Read the model definition and answer for the solid it produces. Units are mm, in the model's axes. Face numbers are marked on the shaded views. A direction names the side the tool comes from. Give positions to 0.01 mm unless a question says otherwise; leave off trailing zeros. Loops run counter-clockwise (first coordinate to the right, second up) from the corner with the lowest first, then second, coordinate; pieces in that order, holes last. Notation, with made-up numbers: (42, 49) - (81, 49) arc R17 ccw to (81, 82) - close; hole circle Ø9 at (86, -29). An arc over 180 degrees is marked (long way). Write item = value, one per line.
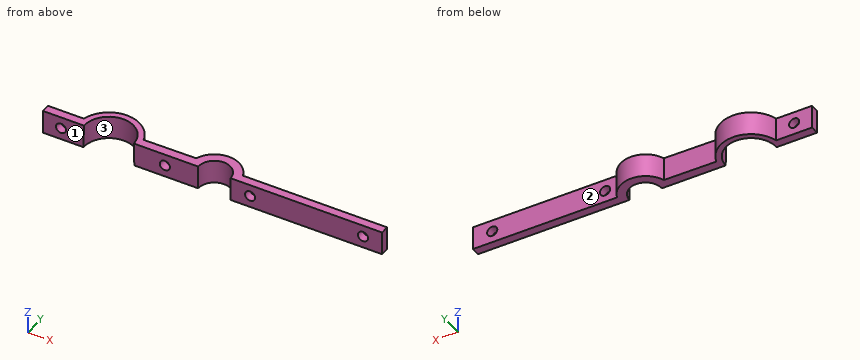
Autodesk Fusion 360 part; units mm, degrees
sketch "Sketch1" plane through (0, 0, 0) normal (0, 0, 1) x (1, 0, 0)
  circle A0 centre (-43.925, 0) radius 12.925
  circle A1 centre (0, 0) radius 10.5
  circle A2 centre (0, 0) radius 6.75
  line L0 (9.8995, 3.5) -> (69.8995, 3.5)
  line L1 (69.8995, 3.5) -> (69.8995, -3.5)
  line L2 (69.8995, -3.5) -> (9.8995, -3.5)
  line L3 (-31.5162, 3.6163) -> (-9.7806, 3.8197)
  line L4 (-31.4507, -3.3834) -> (-10.006, -3.1827)
  line L5 (-56.3671, 3.5) -> (-71.3671, 3.5)
  line L6 (-71.3671, 3.5) -> (-71.3671, -3.5)
  line L7 (-71.3671, -3.5) -> (-56.3671, -3.5)
  line L8 (-43.925, 0) -> (0, 0) construction
  dimension "d1" = 3.5
  dimension "d2" = 3.5
  dimension "d3" = 3.5
  dimension "d4" = 3.5
  dimension "d5" = 3.5
  dimension "d6" = 3.5
  dimension "d7" = 43.925
  dimension "d8" = 60
  dimension "d9" = 15
  dimension "d19" = 25.85
  dimension "d20" = 21
  dimension "d21" = 13.5
extrude "Extrude1" add sketch "Sketch1" along normal mid plane 10
sketch "Sketch4" plane through (0, 3.5, 0) normal (0, 1, 0) x (-1, 0, 0)
  line L0 (71.3671, -5) -> (71.3671, 5)
  line L1 (71.3671, 5) -> (56.3671, 5)
  line L2 (56.3671, 5) -> (56.3671, -5)
  line L3 (56.3671, -5) -> (71.3671, -5)
  circle A0 centre (63.8671, 0) radius 2.125
  line L4 (31.5162, -5) -> (9.7806, -5)
  line L5 (31.5162, 5) -> (31.5162, -5)
  line L6 (9.7806, -5) -> (9.7806, 5)
  dimension "d25" = 4.25
  dimension "d27" = 5
  dimension "d31" = 7.5
  dimension "d32" = 7.5
extrude "Extrude4" cut sketch "Sketch4" along normal up to surface contours A0 end surface through (-31.4507, -3.3834, 0) normal (0.009359, -0.999956, 0) offset 0
sketch "Sketch5" plane through (-0.0366, 3.9109, 0) normal (-0.0094, 1, 0) x (0, 0, 1)
  line L0 (-5, -31.481) -> (5, -31.481)
  line L1 (5, -31.481) -> (5, -9.7444)
  line L2 (5, -9.7444) -> (-5, -9.7444)
  line L3 (-5, -9.7444) -> (-5, -31.481)
  circle A0 centre (0, -20.613) radius 2.125
  dimension "d35" = 4.25
  dimension "d36" = 10.868
  dimension "d37" = 10.8686
  dimension "d38" = 5
extrude "Extrude5" cut sketch "Sketch5" against normal up to surface (7 mm away) contours A0
sketch "Sketch6" plane through (0, 3.5, 0) normal (0, 1, 0) x (-1, 0, 0)
  line L0 (-9.8995, -5) -> (-9.8995, 5)
  line L1 (-9.8995, 5) -> (-69.8995, 5)
  line L2 (-69.8995, 5) -> (-69.8995, -5)
  line L3 (-69.8995, -5) -> (-9.8995, -5)
sketch "Sketch7" plane through (0, 3.5, 0) normal (0, 1, 0) x (-1, 0, 0)
  line L0 (-9.8995, -5) -> (-9.8995, 5) construction
  line L1 (-9.8995, 5) -> (-69.8995, 5) construction
  line L2 (-69.8995, 5) -> (-69.8995, -5) construction
  line L3 (-69.8995, -5) -> (-9.8995, -5) construction
  line L4 (-69.8995, 0) -> (-9.8995, 0) construction
  circle A0 centre (-61.8995, 0) radius 2.125
  circle A1 centre (-14.8995, 0) radius 2.125
  dimension "d41" = 4.25
  dimension "d42" = 4.25
  dimension "d43" = 8
  dimension "d44" = 5
extrude "Extrude6" cut sketch "Sketch7" against normal up to surface (7 mm away)
sketch "Sketch8" plane through (0, 0, 5) normal (0, 0, 1) x (1, 0, 0)
  circle A0 centre (0, 0) radius 6.75
  arc A1 (-31.5162, 3.6163) -> (-56.3671, 3.5) centre (-43.925, 0) ccw
  line L0 (-56.3671, 3.5) -> (-71.3671, 3.5)
  line L1 (-71.3671, 3.5) -> (-71.3671, -3.5)
  line L2 (-71.3671, -3.5) -> (-56.3671, -3.5)
  arc A2 (-56.3671, -3.5) -> (-31.4507, -3.3834) centre (-43.925, 0) ccw
  line L3 (-31.4507, -3.3834) -> (-10.006, -3.1827)
  arc A3 (-10.006, -3.1827) -> (9.8995, -3.5) centre (0, 0) ccw
  line L4 (9.8995, -3.5) -> (69.8995, -3.5)
  line L5 (69.8995, -3.5) -> (69.8995, 3.5)
  line L6 (69.8995, 3.5) -> (9.8995, 3.5)
  arc A4 (9.8995, 3.5) -> (-9.7806, 3.8197) centre (0, 0) ccw
  line L7 (-9.7806, 3.8197) -> (-31.5162, 3.6163)
  circle A5 centre (-43.925, 0) radius 12.925 construction
  circle A6 centre (-43.925, 0) radius 10.37
  dimension "d49" = 20.74
sketch "Sketch9" plane through (0, 0, -5) normal (0, 0, -1) x (-1, 0, 0)
  circle A0 centre (0, 0) radius 6.75
  arc A1 (56.3671, 3.5) -> (31.5162, 3.6163) centre (43.925, 0) ccw
  line L0 (31.5162, 3.6163) -> (9.7806, 3.8197)
  arc A2 (9.7806, 3.8197) -> (-9.8995, 3.5) centre (0, 0) ccw
  line L1 (-9.8995, 3.5) -> (-69.8995, 3.5)
  line L2 (-69.8995, 3.5) -> (-69.8995, -3.5)
  line L3 (-69.8995, -3.5) -> (-9.8995, -3.5)
  arc A3 (-9.8995, -3.5) -> (10.006, -3.1827) centre (0, 0) ccw
  line L4 (10.006, -3.1827) -> (31.4507, -3.3834)
  arc A4 (31.4507, -3.3834) -> (56.3671, -3.5) centre (43.925, 0) ccw
  line L5 (56.3671, -3.5) -> (71.3671, -3.5)
  line L6 (71.3671, -3.5) -> (71.3671, 3.5)
  line L7 (71.3671, 3.5) -> (56.3671, 3.5)
  circle A5 centre (43.925, 0) radius 12.925 construction
  circle A6 centre (43.925, 0) radius 10.6
  dimension "d50" = 21.2
loft "Loft1" cut profiles "Sketch8", "Sketch9" section 1 contours A6 section 2 contours A6
sketch "Sketch3" plane through (0, 0, 0) normal (0, 1, 0) x (1, 0, 0)
  line L0 (-71.3671, 5) -> (-71.3671, -5)
  line L1 (-71.3671, -5) -> (-56.3671, -5)
  line L2 (-56.3671, -5) -> (-56.3671, 5)
  line L3 (-56.3671, 5) -> (-71.3671, 5)
  line L4 (9.8995, 5) -> (9.8995, -5)
  line L5 (9.8995, -5) -> (69.8995, -5)
  line L6 (69.8995, -5) -> (69.8995, 5)
  line L7 (69.8995, 5) -> (9.8995, 5)
  line L8 (-71.3671, 5) -> (69.8995, 5)
  line L9 (69.8995, 5) -> (69.8995, -5)
  line L10 (69.8995, -5) -> (-71.3671, -5)
  line L11 (-71.3671, -5) -> (-71.3671, 5)
  circle A0 centre (-63.8671, 0) radius 2.125
  circle A1 centre (14.8995, 0) radius 2.125
  circle A2 centre (61.8995, 0) radius 2.125
extrude "Extrude3" cut sketch "Sketch3" against normal blind 20 contours L0 L1 L2 L3 L8 L10 L11 | L2 L4 L8 L10 | L4 L5 L6 L7 L8 L9 L10 | A0 | A1 | A2
equation "d2 = d1"
equation "d3 = d1"
equation "d4 = d1"
equation "d5 = d1"
equation "d6 = d1"
equation "d42 = d41"
1) A cutting plane is placed at B-B on x = 30.5. Determine the outline of the cut face in (y, z).
Output:
outline = (0, -5) - (3.5, -5) - (3.5, 5) - (0, 5) - close
2) A cutting plane is placed at D-D on x = 0. Determine the outline of the cut face in (y, z).
Output:
outline = (6.75, -5) - (10.5, -5) - (10.5, 5) - (6.75, 5) - close
3) A tool of negligible diameter and unlimited length cuts with its end or side. For the marked faces 1, 2 and 3, from which of +Z, -Z, +X, -X, +Y, -Y can it reach the whole face along a straight path? Write none if from no direction.
Output:
face_1 = +Z, -Z, +X, -X, -Y
face_2 = +Z, -Z, +X, +Y
face_3 = -Z, -Y
4) Find the intervals of material crossed by probe 1 along X at (y, z) = (7.5, 4.75); probe 2 along X at (y, z) = (7.75, -3.75); probe 3 along Y at (x, z) = (32, 1.5), in increasing order.
Output:
probe_1 = -54.45 to -51.09, -36.76 to -33.4, -7.35 to 7.35
probe_2 = -54.27 to -51.11, -36.74 to -33.58, -7.08 to 7.08
probe_3 = 0 to 3.5
5) Each of these flat-tipped pins is pushed along its axis until it touches: P1, Ø5, axis at x = -63.5, z = -1.5, coming from the +Y side; P2, Ø4, axis at x = -4.5, y = 4.5, coming from the +Z side; P3, Ø3.5, axis at x = 61.9, z = 0, coming from the -Y side. Where does it stop, or does it pass through?
Output:
P1 = 3.5
P2 = 5
P3 = through
6) A cutting plane is placed at A-A on z = 0. Give the number of separate pieces and of enclosed holes in the cut face, then the cut area to 3 significant figures.
Output:
separate_pieces = 4
enclosed_holes = 0
area = 469 mm²
